Build history of the part. All positions in model axes, mm. Round coordinates to 2 decimals unless told otherwise and drop trailing zeros. Loops run counter-clockwise (first coordinate to the right, second up) from the corner with the lowest first, then second, coordinate; pieces in that order, holes last. Notation, with made-up numbers: (-5, 9.25) - (26, 9.25) arc R15 cw to (26, 35.25) - close; hole circle Ø9 at (28, 69.5). An arc over 180 degrees is marked (long way). Use one line per item in the form item = value. Start each with the question number.
Q1. Saw through at C-C (z = -48). Give the cut face in (x, y), then the cut area to 3 significant figures.
Q2. Pin check, flat tips, straight feed: pin 1 (12 mm diameter, centred on y = -18.5, z = 4.5, fed in from -X); pin 2 (4 mm diameter, centred on y = -16, z = -17, fed in from +X); pin 3 (10 mm diameter, centred on x = -25, z = 43, fed in from +Y). Stop position of each tip, or through.
Q3. Saw through at B-B (y = -13.5). Give the cut face in (x, z), then the cut area to 3 significant figures.
Q4. Drill centre lines: line 1 (Z direction, x = -26, y = -48); line 2 (Y direction, x = 31, z = 23.5); line 3 (Z direction, x = 44, y = -32.5). Where is each one in solid material? Low to high.
Q5. Saw through at D-D (x = -47.5). Give the cut face in (y, z).
Q6. Saw through at A-A (x = 4.5). Give the cut face in (y, z), then the cut area to 3 significant figures.
```python
from build123d import *

# Parameters (mm, degrees)
F0_R     = 63.5
F1_DEPTH = 63.5
F2_W     = 209.9135220051
F2_H     = 188.6474490166
F2_R     = 63.5
F3_DEPTH = 63.5
F4_W     = 154.9591273069
F4_H     = 152.5524
F4_R     = 63.5
F5_DEPTH = 63.5


with BuildPart() as f1:
    # F0 (on Front) → F1 (new body, symmetric)
    with BuildSketch(Plane.XZ):
        Circle(F0_R)
    extrude(amount=F1_DEPTH, both=True)

    # F2 (on Top) → F3 (cut, symmetric)
    with BuildSketch(Plane.XY):
        Rectangle(F2_W, F2_H)
        Circle(F2_R, mode=Mode.SUBTRACT)
    extrude(amount=F3_DEPTH, both=True, mode=Mode.SUBTRACT)

    # F4 (on Right) → F5 (cut, symmetric)
    with BuildSketch(Plane.YZ):
        Rectangle(F4_W, F4_H)
        Circle(F4_R, mode=Mode.SUBTRACT)
    extrude(amount=F5_DEPTH, both=True, mode=Mode.SUBTRACT)


solid = f1.part
```
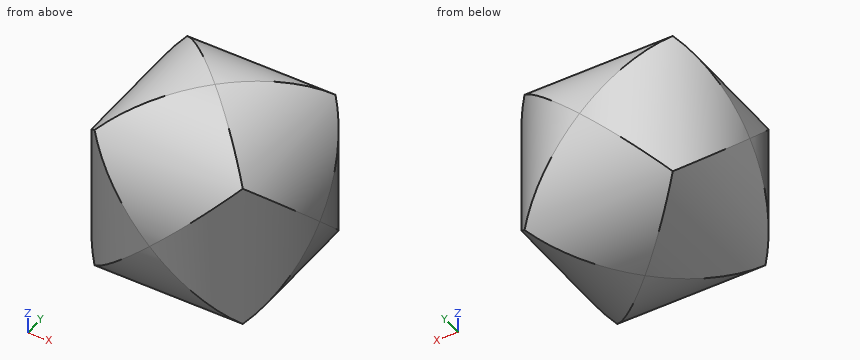
Report:
q1.outline = (-41.57, -41.57) - (41.57, -41.57) - (41.57, 41.57) - (-41.57, 41.57) - close
q1.area = 6,910 mm²
q2.pin_1 = -62.26
q2.pin_2 = 61.66
q2.pin_3 = 50.87
q3.outline = (-62.05, -13.5) arc R63.5 ccw to (-13.5, -62.05) - (13.5, -62.05) arc R63.5 ccw to (62.05, -13.5) - (62.05, 13.5) arc R63.5 ccw to (13.5, 62.05) - (-13.5, 62.05) arc R63.5 ccw to (-62.05, 13.5) - close
q3.area = 12,600 mm²
q4.line_1 = -41.57 to 41.57
q4.line_2 = -55.42 to 55.42
q4.line_3 = -45.78 to 45.78
q5.outline = (-42.14, -42.14) - (42.14, -42.14) - (42.14, 42.14) - (-42.14, 42.14) - close
q6.outline = (-63.34, -4.5) arc R63.5 ccw to (-4.5, -63.34) - (4.5, -63.34) arc R63.5 ccw to (63.34, -4.5) - (63.34, 4.5) arc R63.5 ccw to (4.5, 63.34) - (-4.5, 63.34) arc R63.5 ccw to (-63.34, 4.5) - close
q6.area = 12,700 mm²
